Verification items for the finished model (mm, model axes). A direction names the side the tool comes from. Give positions to 0.01 mm unless a question says otherwise; leave off trailing zeros. Order: outer loops, then holes, each group sorted by start corner. A loop starts at its lowest first (then second) coordinate and runs counter-clockwise, first axis right, second up. Notation, with made-up numbers: M -15,-4 L 34,-4 A36 cw 34,30 Z; hole C 37,-32 d7. An arc over 180 degrees is marked long. Answer as a JSON object with one key per item and string values.
```python
from build123d import *

# Parameters (mm, degrees)
CORTAR_EXTRUIR1_DEPTH   = 9
CROQUIS5_R              = 4
CORTAR_EXTRUIR3_DEPTH   = 27
CROQUIS6_R              = 2
CORTAR_EXTRUIR4_DEPTH   = 10
CROQUIS7_R              = 2
SALIENTE_EXTRUIR1_DEPTH = 3.5
CROQUIS8_R              = 7
CROQUIS8_R_2            = 2
CORTAR_EXTRUIR5_DEPTH   = 3.5


with BuildPart() as part:
    # Croquis1 → Revolución1 (revolve)
    with BuildSketch(Plane(origin=(0, 0, 0), x_dir=(1, 0, 0), z_dir=(0, 1, 0))):
        Polygon((0, 1.5), (0, -9.5), (7, -9.5), (7, -13), (12.5, -13), (27.5, -13), (27.5, -7.5), (20, -7.5), (20, -2.5), (27.5, -2.5), (27.5, 2.5), (20, 2.5), (20, 7.5), (27.5, 7.5), (27.5, 13), (12.5, 13), (12.5, 6.5), (7.5, 1.5), align=None)
    revolve(axis=Axis((0, 0, 0), (0, 0, -1)))

    # Croquis2 → Cortar-Extruir1 (cut)
    with BuildSketch(Plane(origin=(0, 0, -1.5), x_dir=(-1, 0, 0), z_dir=(0, 0, -1))):
        Polygon((7.505553499, 0), (3.75277675, 6.5), (-3.75277675, 6.5), (-7.505553499, 0), (-3.75277675, -6.5), (3.75277675, -6.5), align=None)
    extrude(amount=-CORTAR_EXTRUIR1_DEPTH, mode=Mode.SUBTRACT)

    # Croquis5 → Cortar-Extruir3 (cut, through all)
    with BuildSketch(Plane.XY.offset(13)):
        with Locations((0, 24.5)):
            Circle(CROQUIS5_R)
        with Locations((12.25, 21.217622393)):
            Circle(CROQUIS5_R)
        with Locations((21.217622393, 12.25)):
            Circle(CROQUIS5_R)
        with Locations((24.5, 0)):
            Circle(CROQUIS5_R)
        with Locations((21.217622393, -12.25)):
            Circle(CROQUIS5_R)
        with Locations((12.25, -21.217622393)):
            Circle(CROQUIS5_R)
        with Locations((0, -24.5)):
            Circle(CROQUIS5_R)
        with Locations((-12.25, -21.217622393)):
            Circle(CROQUIS5_R)
        with Locations((-21.217622393, -12.25)):
            Circle(CROQUIS5_R)
        with Locations((-24.5, 0)):
            Circle(CROQUIS5_R)
        with Locations((-21.217622393, 12.25)):
            Circle(CROQUIS5_R)
        with Locations((-12.25, 21.217622393)):
            Circle(CROQUIS5_R)
    extrude(amount=-CORTAR_EXTRUIR3_DEPTH, mode=Mode.SUBTRACT)

    # Croquis6 → Cortar-Extruir4 (cut)
    with BuildSketch(Plane(origin=(0, 0, 7.5), x_dir=(-1, 0, 0), z_dir=(0, 0, -1))):
        Circle(CROQUIS6_R)
    extrude(amount=-CORTAR_EXTRUIR4_DEPTH, mode=Mode.SUBTRACT)

    # Croquis7 → Saliente-Extruir1 (add)
    with BuildSketch(Plane(origin=(0, 0, 7.5), x_dir=(-1, 0, 0), z_dir=(0, 0, -1))):
        Polygon((3.75277675, -6.5), (7.505553499, 0), (3.75277675, 6.5), (-3.75277675, 6.5), (-7.505553499, 0), (-3.75277675, -6.5), align=None)
        Circle(CROQUIS7_R, mode=Mode.SUBTRACT)
    extrude(amount=SALIENTE_EXTRUIR1_DEPTH)

    # Croquis8 → Cortar-Extruir5 (cut)
    with BuildSketch(Plane.XY.offset(9.5)):
        Circle(CROQUIS8_R)
        Circle(CROQUIS8_R_2, mode=Mode.SUBTRACT)
    extrude(amount=-CORTAR_EXTRUIR5_DEPTH, mode=Mode.SUBTRACT)


solid = part.part
```
Q1. Section check B-B on x = -14. Record the cut outline in (y, z).
Resolved:
{"outline": "M -17.62,-13 L 17.62,-13 L 17.62,-7.5 L 14.28,-7.5 L 14.28,-2.5 L 17.62,-2.5 L 17.62,2.5 L 14.28,2.5 L 14.28,7.5 L 17.62,7.5 L 17.62,13 L -17.62,13 L -17.62,7.5 L -14.28,7.5 L -14.28,2.5 L -17.62,2.5 L -17.62,-2.5 L -14.28,-2.5 L -14.28,-7.5 L -17.62,-7.5 Z"}
Q2. Gauge pin test, flat ends, axial feed: pin 1 Ø0.5 at (x, y) = (0.5, -7) entering from -Z; pin 2 Ø1 at (y, z) = (-2, 1.5) entering from +X; pin 3 Ø5 at (y, z) = (0, 3) entering from -X; pin 4 Ø7 at (x, y) = (0, 24.5) entering from +Z. Record the tip position at first contact, or that the pin passes through.
Resolved:
{"pin 1": "stops at z = -1.5", "pin 2": "stops at x = 21.38", "pin 3": "stops at x = -21.34", "pin 4": "passes through"}
Q3. Section check C-C on y = -18. Count the separate pieces of the cut face and the enclosed holes in it, then the cut area to 3 significant figures.
Resolved:
{"separate pieces": "7", "enclosed holes": "0", "area": "688 mm²"}
Q4. Tool access check on faces 1 (the face through (19.49, -19.4, 10.21)), 2 (the face through (-6, -4, -1.5)). Record the directions out of +Z, -Z, +X, -X, +Y, -Y that give a thin tool (end or side, any length) a straight path to the whole face; none if there is none.
Resolved:
{"face 1": "+Z, -Z, +X, -Y", "face 2": "-Z"}
Q5. Release check for a two-part mould opening along Y. For faces 3 (the face through (26.547, 7.177, 10.212)), 4 (the face through (-14.3, -14.3, 7.5)), 5 (the face through (-5.6, -3.3, 1.2)) record: +Y half, -Y half, draft (parallel to the pull), parting line (faces both ways), or undercut.
Resolved:
{"face 3": "+Y half", "face 4": "draft", "face 5": "undercut"}
Q6. Material ranges on L1, parallel to Z at x = -13, y = 16; L2, parallel to X at y = -10, z = -1.25; L3, parallel to X at y = -11, z = -2.25, recorded low to high.
Resolved:
{"L1": "z = -13 to -7.5, -2.5 to 2.5, 7.5 to 13", "L2": "x = -25.62 to -24.52, -17.91 to 17.91, 24.52 to 25.62", "L3": "x = -25.2 to -25.02, -17.42 to 17.42, 25.02 to 25.2"}
Q7. Section check A-A on z = -8.5. Record the cut outline in (x, y), then the cut area to 3 significant figures.
Resolved:
{"outline": "M -27.36,-2.8 A27.5 ccw -25.09,-11.25 A4 cw long -22.29,-16.1 A27.5 ccw -16.1,-22.29 A4 cw long -11.25,-25.09 A27.5 ccw -2.8,-27.36 A4 cw long 2.8,-27.36 A27.5 ccw 11.25,-25.09 A4 cw long 16.1,-22.29 A27.5 ccw 22.29,-16.1 A4 cw long 25.09,-11.25 A27.5 ccw 27.36,-2.8 A4 cw long 27.36,2.8 A27.5 ccw 25.09,11.25 A4 cw long 22.29,16.1 A27.5 ccw 16.1,22.29 A4 cw long 11.25,25.09 A27.5 ccw 2.8,27.36 A4 cw long -2.8,27.36 A27.5 ccw -11.25,25.09 A4 cw long -16.1,22.29 A27.5 ccw -22.29,16.1 A4 cw long -25.09,11.25 A27.5 ccw -27.36,2.8 A4 cw long Z; hole C 0,0 d25", "area": "1,330 mm²"}
